```python
from build123d import *

# Parameters (mm, degrees)
SKETCH_1_W          = 10
SKETCH_1_H          = 3
SKETCH_1_W_2        = 3
SKETCH_1_H_2        = 10
EXTRUDE_1_DEPTH     = 3
SKETCH_2_W          = 14
SKETCH_2_H          = 7
CUT_EXTRUDE_1_DEPTH = 10


with BuildPart() as part:
    # 草图1 → 凸台-拉伸1 (new body)
    with BuildSketch(Plane.XY):
        Polygon((-5, 22.5), (-5, 25.5), (5, 25.5), (5, 22.5), (15, 22.5), (15, 25.5), (25, 25.5), (25, 22.5), (32.5, 22.5), (32.5, -22.5), (-32.5, -22.5), (-32.5, 22.5), (-25, 22.5), (-25, 25.5), (-15, 25.5), (-15, 22.5), align=None)
        with Locations((-7.5, -19)):
            Rectangle(SKETCH_1_W, SKETCH_1_H, mode=Mode.SUBTRACT)
        with Locations((-22.5, -19)):
            Rectangle(SKETCH_1_W, SKETCH_1_H, mode=Mode.SUBTRACT)
        with Locations((7.5, -19)):
            Rectangle(SKETCH_1_W, SKETCH_1_H, mode=Mode.SUBTRACT)
        with Locations((22.5, -19)):
            Rectangle(SKETCH_1_W, SKETCH_1_H, mode=Mode.SUBTRACT)
        with Locations((-29, -7.5)):
            Rectangle(SKETCH_1_W_2, SKETCH_1_H_2, mode=Mode.SUBTRACT)
        with Locations((-29, 12.5)):
            Rectangle(SKETCH_1_W_2, SKETCH_1_H_2, mode=Mode.SUBTRACT)
        with Locations((29, -7.5)):
            Rectangle(SKETCH_1_W_2, SKETCH_1_H_2, mode=Mode.SUBTRACT)
        with Locations((29, 12.5)):
            Rectangle(SKETCH_1_W_2, SKETCH_1_H_2, mode=Mode.SUBTRACT)
    extrude(amount=EXTRUDE_1_DEPTH)

    # 草图2 → 切除-拉伸1 (cut)
    with BuildSketch(Plane.XY.offset(3)):
        with Locations((-8.812746432, 1)):
            Rectangle(SKETCH_2_W, SKETCH_2_H)
    extrude(amount=-CUT_EXTRUDE_1_DEPTH, mode=Mode.SUBTRACT)


solid = part.part
```
Design review of the part built by this model. Coordinates are the model's own, in mm. A direction names the side the tool comes from. Coordinates: 2 decimals unless noted, no trailing zeros. Order: outer loops, then holes, each group sorted by start corner. A loop starts at its lowest first (then second) coordinate and runs counter-clockwise, first axis right, second up.
1) Take a section at D-D, the plane z = 1.35. State how many separate pieces and enclosed holes the cut face has, and give its area (3 significant figures).
2) Take a section at B-B, the plane y = -1. Give the boundary of the cut face in (x, z).
3) Take a section at C-C, the plane y = -8. Give the boundary of the cut face in (x, z).
4) Take a section at A-A, the plane x = -20.5. Give the boundary of the cut face in (y, z).
5) Clearance check with flat-ended pins moving along their axes: pin 1 (1.5 mm diameter, centred on y = 24, z = 2, fed in from -X); pin 2 (0.9 mm diameter, centred on x = -8.5, z = 2, fed in from +Y). State where each tip first meets the part, or that it passes through.
6) Mouldability with a two-part tool opening along X and no side actions: class faces 6 (the flat face through (32.5, 0, 1)), 7 (the flat face through (29, 7.5, 1)), 8 (the flat face through (0, 2, 3)) as +X half, -X half, draft (parallel to the pull), parting line (faces both ways), or undercut.
7) For faces 1 (the flat face through (20, 25.5, 1)), 2 (the flat face through (29, 22.5, 1)), 3 (the flat face through (10, 22.5, 1)), 4 (the flat face through (-8, -17.5, 1)), 5 (the flat face through (-25, 24, 1)), list the 3-axis set-ups (+Z, -Z, +X, -X, +Y, -Y) from which the entire face can be reached by the end or side of a thin tool; tool diameter is ignored.
8) Wall thickness on line 1 along Y through (x, z) = (-3, 1); line 2 along Y through (x, z) = (-9.5, 1.6); line 3 along X through (y, z) = (-8.5, 1.55): over which ranges is each line inside the solid? List them lowest first.
Returned:
1. separate pieces: 1
1. enclosed holes: 9
1. area: 2,680 mm2
2. outline: (-32.5, 0) - (-15.81, 0) - (-15.81, 3) - (-32.5, 3) - close; (-1.81, 0) - (32.5, 0) - (32.5, 3) - (-1.81, 3) - close
3. outline: (-32.5, 0) - (-30.5, 0) - (-30.5, 3) - (-32.5, 3) - close; (-27.5, 0) - (27.5, 0) - (27.5, 3) - (-27.5, 3) - close; (30.5, 0) - (32.5, 0) - (32.5, 3) - (30.5, 3) - close
4. outline: (-22.5, 0) - (-20.5, 0) - (-20.5, 3) - (-22.5, 3) - close; (-17.5, 0) - (25.5, 0) - (25.5, 3) - (-17.5, 3) - close
5. pin 1: stops at x = -25
5. pin 2: stops at y = 22.5
6. face 6: +X half
6. face 7: undercut
6. face 8: draft
7. face 1: +Z, -Z, +X, -X, +Y
7. face 2: +Z, -Z, +X, +Y
7. face 3: +Z, -Z, +Y
7. face 4: +Z, -Z
7. face 5: +Z, -Z, -X, +Y
8. line 1: y = -22.5 to -20.5, -17.5 to -2.5, 4.5 to 25.5
8. line 2: y = -22.5 to -20.5, -17.5 to -2.5, 4.5 to 22.5
8. line 3: x = -32.5 to -30.5, -27.5 to 27.5, 30.5 to 32.5
